from build123d import *

# Parameters (mm, degrees)
F0_R     = 1.5875
F1_DEPTH = 34.29
F2_R     = 5.08


with BuildPart() as f1:
    # F0 (on Front) → F1 (new body)
    with BuildSketch(Plane.XZ):
        Polygon((29.623586, 16.249556), (12.24797, 31.489556), (-10.858607, 31.995243), (-28.884321, 17.53), (-33.39474, -5.137725), (-22.27939, -25.401451), (-0.739265, -33.779556), (21.14677, -26.351831), (33.137997, -6.593792), align=None)
        Circle(F0_R, mode=Mode.SUBTRACT)
    extrude(amount=-F1_DEPTH)

    # F2
    f2_edges = [f1.edges().sort_by_distance(p)[0] for p in [
        (-31.139531, 0, 6.196138),
        (-27.837065, 0, -15.269588),
        (-19.871464, 0, 24.762621),
        (0.694682, 0, 31.742399),
        (20.935778, 0, 23.869556),
        (31.380791, 0, 4.827882),
        (27.142383, 0, -16.472812),
        (10.203753, 0, -30.065694),
        (-11.509327, 0, -29.590503),
        (27.142383, 34.29, -16.472812),
        (31.380791, 34.29, 4.827882),
        (20.935778, 34.29, 23.869556),
        (0.694682, 34.29, 31.742399),
        (-19.871464, 34.29, 24.762621),
        (-31.139531, 34.29, 6.196138),
        (-27.837065, 34.29, -15.269588),
        (-11.509327, 34.29, -29.590503),
        (10.203753, 34.29, -30.065694),
    ]]
    fillet(f2_edges, radius=F2_R)


solid = f1.part
Input: part model. Units: mm. Frame: model coordinates. A direction names the side the tool comes from. Give positions to 0.01 mm unless a question says otherwise; leave off trailing zeros. Write each loop counter-clockwise with the first axis right and the second up, starting at its lowest first coordinate (ties: lowest second). Pieces come first, ordered by that corner, then holes.
Q1. First-contact query: P1, Ø12, axis at y = 12, z = 16, coming from the -X side; P2, Ø10, axis at x = -4.5, y = 24, coming from the +Z side; P3, Ø12, axis at x = 3.5, y = 4, coming from the +Z side. Flat tips, straight axial feed; report the tip coordinate or a pass-through.
Q2. Set-up query: faces 1 (the face through (31.4, 17, 4.7)), 2 (the face through (0.5, 32.76, 30.3)). Return all of +Z, -Z, +X, -X, +Y, -Y with unobstructed straight access to the full face (end or side cutting, diameter ignored); none if empty.
Q3. Material intervals for probe 1 along Z at (x, y) = (0, 26); probe 2 along X at (y, z) = (30.5, 0.5); probe 3 along Z at (x, y) = (-1, 2.5), sorted ascending.
Q4. Section A-A, the plane y = 16.5. Output: boundary loops of the cut face in (x, z) (1 decimal), plus the area to 3 significant figures.
Filled in:
1. P1: stops at x = -30.38
1. P2: stops at z = 31.97
1. P3: stops at z = 31.81
2. face 1: +Z, +X, +Y, -Y
2. face 2: +Z, +X, +Y
3. probe 1: z = -33.53 to -1.59, 1.59 to 31.76
3. probe 2: x = -32.1 to -1.51, 1.51 to 31.88
3. probe 3: z = -32.92 to -1.23, 1.23 to 31.08
4. outline: (-33.4, -5.1) - (-22.3, -25.4) - (-0.7, -33.8) - (21.1, -26.4) - (33.1, -6.6) - (29.6, 16.2) - (12.2, 31.5) - (-10.9, 32) - (-28.9, 17.5) - close; hole circle Ø3.2 at (0, 0)
4. area: 3,290 mm2
